```python
from build123d import *

# Parameters (mm, degrees)
SKETCH_W        = 130.707065
SKETCH_H        = 59.583364
SKETCH_W_2      = 30
SKETCH_H_2      = 39.583364
PAD_DEPTH       = 40
SKETCH001_R     = 9
POCKET_DEPTH    = 32
SKETCH002_R     = 9
POCKET001_DEPTH = 16
SKETCH003_R     = 9
POCKET002_DEPTH = 21
SKETCH004_R     = 9
POCKET003_DEPTH = 23


with BuildPart() as part:
    # Sketch → Pad (new body)
    with BuildSketch(Plane.XY):
        with Locations((-4.646459, 9.990193)):
            Rectangle(SKETCH_W, SKETCH_H)
        with Locations((-44.357391, 9.990193)):
            Rectangle(SKETCH_W_2, SKETCH_H_2, mode=Mode.SUBTRACT)
        with Locations((-5.023146, 10.351241)):
            Rectangle(SKETCH_W_2, SKETCH_H_2, mode=Mode.SUBTRACT)
        with Locations((35.101015, 9.990193)):
            Rectangle(SKETCH_W_2, SKETCH_H_2, mode=Mode.SUBTRACT)
    extrude(amount=PAD_DEPTH)

    # Sketch001 (on Face4 of Pad) → Pocket (cut)
    with BuildSketch(Plane(origin=(-69.999992, 0, 0), x_dir=(0, -1, 0), z_dir=(-1, 0, 0))):
        with Locations((-10.001616, 19.98172)):
            Circle(SKETCH001_R)
    extrude(amount=-POCKET_DEPTH, mode=Mode.SUBTRACT)

    # Sketch002 (on Face17 of Pocket) → Pocket001 (cut)
    with BuildSketch(Plane(origin=(-29.357391, 0, 0), x_dir=(0, -1, 0), z_dir=(-1, 0, 0))):
        with Locations((-10.001346, 19.991329)):
            Circle(SKETCH002_R)
    extrude(amount=-POCKET001_DEPTH, mode=Mode.SUBTRACT)

    # Sketch003 (on Face13 of Pocket001) → Pocket002 (cut)
    with BuildSketch(Plane(origin=(9.976854, 0, 0), x_dir=(0, -1, 0), z_dir=(-1, 0, 0))):
        with Locations((-9.927585, 19.937319)):
            Circle(SKETCH003_R)
    extrude(amount=-POCKET002_DEPTH, mode=Mode.SUBTRACT)

    # Sketch004 (on Face9 of Pocket002) → Pocket003 (cut)
    with BuildSketch(Plane(origin=(50.101015, 0, 0), x_dir=(0, -1, 0), z_dir=(-1, 0, 0))):
        with Locations((-9.980604, 20.028202)):
            Circle(SKETCH004_R)
    extrude(amount=-POCKET003_DEPTH, mode=Mode.SUBTRACT)


solid = part.part
```
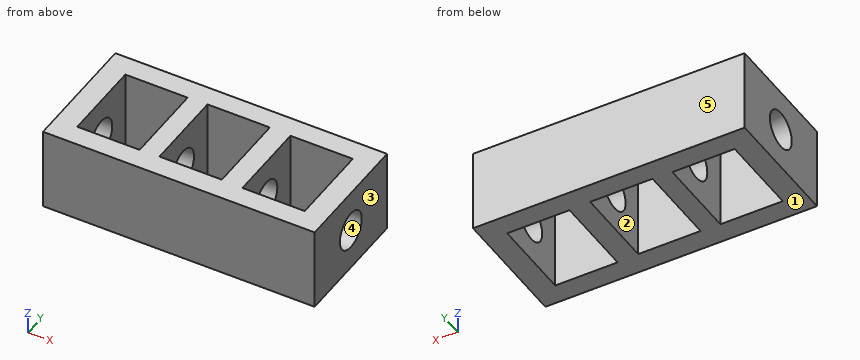
Work out the finished part from the listing and answer in its coordinate system (mm). Face numbers are marked on the shaded views. A direction names the side the tool comes from. Give positions to 0.01 mm unless a question says otherwise; leave off trailing zeros. Loops run counter-clockwise (first coordinate to the right, second up) from the corner with the lowest first, then second, coordinate; pieces in that order, holes last. Notation, with made-up numbers: (51.25, -18) -> (109.25, -18) arc R16 ccw to (109.25, 0) -> close; hole circle Ø3 at (-11, 81). An arc over 180 degrees is marked (long way). Put each result on its own line as item: value. Start each with the question number.
Item 1: The part is cut by section C-C (z = 34). Give the vertices of the cut face in (x, y).
Item 2: Which of the six approach directions +Z, -Z, +X, -X, +Y, -Y give full straight-line access (tool end or side, diameter ignored) to the marked faces 1 and 2?
Item 3: The part is cut by section A-A (x = 31). Give the vertices of the cut face in (y, z).
Item 4: The part is cut by section B-B (y = 22). Give the vertices of the cut face in (x, z).
Item 5: This flat-tipped pin is pushed along its axis until it touches: P1, Ø14.5, axis at y = 9.93, z = 19.94, coming from the -X side. Where does it stop, or does it pass through?
Item 6: The mould has two halves that part along Y. Classify the marked faces 3, 4 and 5: released by +Y, released by -Y, zero draft, split by the parting line, or undercut.
Item 7: Find the intervals of material crossed by L1, parallel to X at y = 24, z = 4; L2, parallel to Y at x = 6, z = 24; L3, parallel to Y at x = 50, z = 38, in increasing order. Write a range as [from, to].
Answers below:
1. outline: (-70, -19.8) -> (60.71, -19.8) -> (60.71, 39.78) -> (-70, 39.78) -> close; hole (-59.36, -9.8) -> (-29.36, -9.8) -> (-29.36, 29.78) -> (-59.36, 29.78) -> close; hole (-20.02, -9.44) -> (9.98, -9.44) -> (9.98, 30.14) -> (-20.02, 30.14) -> close; hole (20.1, -9.8) -> (50.1, -9.8) -> (50.1, 29.78) -> (20.1, 29.78) -> close
2. face 1: -Z, +X, -X, +Y, -Y
2. face 2: +Z, -Z
3. outline: (-19.8, 0) -> (-9.8, 0) -> (-9.8, 40) -> (-19.8, 40) -> close; (29.78, 0) -> (39.78, 0) -> (39.78, 40) -> (29.78, 40) -> close
4. outline: (-70, 0) -> (-59.36, 0) -> (-59.36, 40) -> (-70, 40) -> close; (-29.36, 0) -> (-20.02, 0) -> (-20.02, 40) -> (-29.36, 40) -> close; (9.98, 0) -> (20.1, 0) -> (20.1, 40) -> (9.98, 40) -> close; (50.1, 0) -> (60.71, 0) -> (60.71, 40) -> (50.1, 40) -> close
5. P1: through
6. face 3: zero draft
6. face 4: undercut
6. face 5: released by +Y
7. L1: [-70, -59.36], [-29.36, -20.02], [9.98, 20.1], [50.1, 60.71]
7. L2: [-19.8, -9.44], [30.14, 39.78]
7. L3: [-19.8, -9.8], [29.78, 39.78]
